Geometry check sheet. Reference: the model listing, model coordinates, mm. Round coordinates to 2 decimals unless told otherwise and drop trailing zeros. One line per item, written item: value. Start each with the question number.
1. Depth check by flat-ended pin: P1, Ø4, axis at x = 50.5, z = -14, coming from the -Y side; P2, Ø2, axis at x = -32, y = -8.5, coming from the -Z side; P3, Ø4, axis at x = 0, y = -46.5, coming from the +Z side; P4, Ø20.5, axis at x = 0, z = 0, coming from the -Y side. Enter the tip coordinate at first touch or a pass-through.
2. Release check for a two-part mould opening along X. For faces 1 (the cylindrical face through (12.114, 41.664, 3.815)), 2 (the cylindrical face through (43.42, -2.75, -12.4)) record: pulls with the +X half, pulls with the -X half, needs draft (parallel to the pull), parting line crosses it, or undercut.
3. Section check A-A (x = -4.5). Count the separate pieces of the cut face and the enclosed holes in it, and give its area (3 significant figures).
4. Scan lines: probe 1 along X at (y, z) = (53, -4); probe 2 along Y at (x, z) = (-25.5, 11); probe 3 along X at (y, z) = (0, 41.5). Record each from-to range of solid material in increasing order. Write a range as [from, to].
from build123d import *

# Parameters (mm, degrees)
F2_R     = 12.7
F3_DEPTH = 88.9
F4_R     = 12.7
F5_DEPTH = 88.9
F6_R     = 12.7
F7_DEPTH = 88.9


with BuildPart() as f1:
    # F0 (on Top) → F1 (revolve)
    with BuildSketch(Plane.XY):
        with BuildLine():
            Line((-74.395262, 0), (78.004738, 0))
            ThreePointArc((78.004738, 0), (1.804738, 76.058195), (-74.395262, 0))
        make_face()
    revolve(axis=Axis((1.804738, 0, 0), (1, 0, 0)))

    # F2 (on Top) → F3 (cut, symmetric)
    with BuildSketch(Plane.XY):
        Circle(F2_R)
    extrude(amount=F3_DEPTH, both=True, mode=Mode.SUBTRACT)

    # F4 (on Right) → F5 (cut, symmetric)
    with BuildSketch(Plane.YZ):
        Circle(F4_R)
    extrude(amount=F5_DEPTH, both=True, mode=Mode.SUBTRACT)

    # F6 (on Front) → F7 (cut, symmetric)
    with BuildSketch(Plane.XZ):
        Circle(F6_R)
    extrude(amount=F7_DEPTH, both=True, mode=Mode.SUBTRACT)


solid = f1.part
Result sheet:
1. P1: stops at y = -58.49
1. P2: stops at z = -68.12
1. P3: stops at z = 61.66
1. P4: passes through
2. face 1: undercut
2. face 2: needs draft
3. separate pieces: 4
3. enclosed holes: 0
3. area: 11,400 mm2
4. probe 1: x = [-52.66, -12.05], [12.05, 56.27]
4. probe 2: y = [-70.14, -6.35], [6.35, 70.14]
4. probe 3: x = [-62.01, -12.7], [12.7, 65.62]
